Model file for the job. Use its own axes, mm. Coordinates: 2 decimals unless noted, no trailing zeros. Write each loop counter-clockwise with the first axis right and the second up, starting at its lowest first coordinate (ties: lowest second). Pieces come first, ordered by that corner, then holes. Notation, with made-up numbers: M -32.5,8.25 L -5.5,8.25 A14 cw -5.5,20.25 Z; hole C 14,-6 d6. An arc over 180 degrees is marked long. One line per question, with ' | ' between items. Start each with the question number.
(1) Cut at A-A (y = 2.75). Write the cut outline in (x, z), plus the area to 3 significant figures.
(2) Cut at B-B (z = -0.8). Write the cut outline in (x, y).
(3) Wall check: probe 1 along X at (y, z) = (0.6, 1.85); probe 2 along X at (y, z) = (2.6, 1.15); probe 3 along Z at (x, y) = (-3.25, 2.05). Give the ranges that are in metal, low to high.
(4) Cut at C-C (z = 0.8). Write the cut outline in (x, y), plus the area to 3 significant figures.
Solid Edge part; units mm, degrees
sketch "Sketch1" plane through (0, 0, 0) normal (0, -1, 0) x (1, 0, 0)
  line L0 (-20.6338, -1.25) -> (-3.6338, -1.25)
  line L1 (-3.6338, -1.25) -> (-2.5849, 0)
  line L2 (-2.1861, 3.5) -> (-2.5849, 0)
  line L3 (-2.1861, 3.5) -> (-20.6338, 3.5)
  line L4 (-20.6338, 3.5) -> (-20.6338, -1.25)
extrude "Protrusion1" add sketch "Sketch1" against normal blind 3
properties material "Stainless Steel, 420"
Filled in:
1) outline: M -20.63,-1.25 L -3.63,-1.25 L -2.58,0 L -2.19,3.5 L -20.63,3.5 Z | area: 85.8 mm²
2) outline: M -20.63,0 L -3.26,0 L -3.26,3 L -20.63,3 Z
3) probe 1: -20.63 to -2.37 | probe 2: -20.63 to -2.45 | probe 3: -0.79 to 3.5
4) outline: M -20.63,0 L -2.49,0 L -2.49,3 L -20.63,3 Z | area: 54.4 mm²
